```python
from build123d import *

# Parameters (mm, degrees)
SKETCH_1_W                  = 320
SKETCH_1_H                  = 210
EXTRUDE_1_DEPTH             = 10
HOLE_WIZARD_M41_D           = 3.3
HOLE_WIZARD_M41_DEPTH       = 11.5
HOLE_WIZARD_M41_CSINK_D     = 4.05
HOLE_WIZARD_M41_CSINK_ANGLE = 120
HOLE_WIZARD_M41_TIP         = 0.991420021


with BuildPart() as part:
    # Эскиз1 → Бобышка-Вытянуть1 (new body)
    with BuildSketch(Plane.XY):
        with Locations((160, 105)):
            Rectangle(SKETCH_1_W, SKETCH_1_H)
    extrude(amount=EXTRUDE_1_DEPTH)

    # Отверстие обработанное метчиком M41
    with Locations(Plane(origin=(0, 0, 0), x_dir=(-1, 0, 0), z_dir=(0, 0, -1))):
        with Locations((-22.625631329, 22.625631329), (-47.374368671, 22.625631329), (-47.374368671, 47.374368671), (-22.625631329, 47.374368671), (-297.374368671, 47.374368671), (-272.625631329, 47.374368671), (-272.625631329, 22.625631329), (-297.374368671, 22.625631329), (-22.625631329, 162.625631329), (-47.374368671, 162.625631329), (-47.374368671, 187.374368671), (-22.625631329, 187.374368671), (-297.374368671, 187.374368671), (-272.625631329, 187.374368671), (-272.625631329, 162.625631329), (-297.374368671, 162.625631329)):
            CounterSinkHole(HOLE_WIZARD_M41_D / 2, HOLE_WIZARD_M41_CSINK_D / 2, depth=HOLE_WIZARD_M41_DEPTH, counter_sink_angle=HOLE_WIZARD_M41_CSINK_ANGLE)
            with Locations((0, 0, -(HOLE_WIZARD_M41_DEPTH + HOLE_WIZARD_M41_TIP / 2))):  # 118° drill point
                Cone(0, HOLE_WIZARD_M41_D / 2, HOLE_WIZARD_M41_TIP, mode=Mode.SUBTRACT)


solid = part.part
```
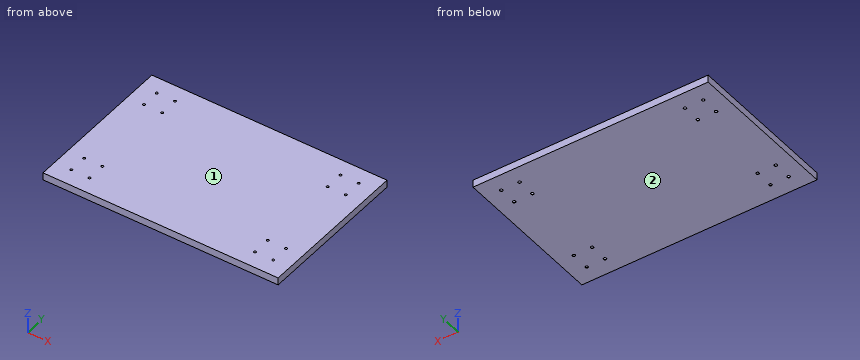
For this review, take the finished solid that the model builds, in its own axes (mm). Face numbers are marked on the shaded views. Give positions to 0.01 mm unless a question says otherwise; leave off trailing zeros. Answer as a JSON object with one key per item and string values. Group by question number.
Item 1: For probe 1 along Y at (x, z) = (47, 4.75); probe 2 along Y at (x, z) = (298.5, 6); probe 3 along X at (y, z) = (164, 5), list the stretches that pass through material, from the lowest coordinate up. Write a range as [from, to].
Item 2: Draft analysis for pull direction Z (two halves, no side actions). For the marked faces 1 and 2, state which applies: +Z half, -Z half, draft (parallel to the pull), parting line (faces both ways), or undercut.
Item 3: For pin 1 Ø5 at (y, z) = (162.5, 6.5) entering from -X; pin 2 Ø3 at (x, y) = (47.37, 187.37) entering from -Z, all flat-tipped, find the tip position at first contact; note any pin that passes through.
Check result:
{
 "1": {"probe 1": "y = [0, 21.02], [24.23, 45.77], [48.98, 161.02], [164.23, 185.77], [188.98, 210]", "probe 2": "y = [0, 21.42], [23.83, 46.17], [48.58, 161.42], [163.83, 186.17], [188.58, 210]", "probe 3": "x = [0, 21.71], [23.54, 46.46], [48.29, 271.71], [273.54, 296.46], [298.29, 320]"},
 "2": {"face 1": "+Z half", "face 2": "-Z half"},
 "3": {"pin 1": "stops at x = 0", "pin 2": "passes through"}
}
